Geometry: final body of the model. Coordinates: model frame, mm. A direction names the side the tool comes from. Round coordinates to 2 decimals unless told otherwise and drop trailing zeros. Loops run counter-clockwise (first coordinate to the right, second up) from the corner with the lowest first, then second, coordinate; pieces in that order, holes last. Notation, with made-up numbers: (46.5, -29) - (63.5, -29) arc R31 ccw to (63.5, 6) - close; hole circle Ø11 at (70, -21.75). An arc over 180 degrees is marked (long way). Answer in a Markdown table with one row per item. Add a question column.
from build123d import *

# Parameters (mm, degrees)
SKETCH1_R           = 2.286
SKETCH1_R_2         = 1.181
BOSS_EXTRUDE1_DEPTH = 6.35
SKETCH1_3_R         = 2.286
SKETCH1_3_R_2       = 1.181
CUT_EXTRUDE1_DEPTH  = 3.175


with BuildPart() as part:
    # Sketch1 → Boss-Extrude1 (new body)
    # profile 1 of 3: a face of its own
    with BuildSketch(Plane.XY):
        with BuildLine():
            Line((399.033701588, 239.383854223), (443.033701589, 239.383854223))
            ThreePointArc((443.033701589, 239.383854223), (444.447915151, 239.969640661), (445.033701588, 241.383854223))
            Line((445.033701588, 241.383854223), (445.033701588, 251.383854223))
            ThreePointArc((445.033701588, 251.383854223), (444.447915152, 252.798067786), (443.033701589, 253.383854224))
            Line((443.033701589, 253.383854224), (399.033701588, 253.383854224))
            ThreePointArc((399.033701588, 253.383854224), (397.619488025, 252.798067787), (397.033701588, 251.383854224))
            Line((397.033701588, 251.383854224), (397.033701588, 241.383854224))
            ThreePointArc((397.033701588, 241.383854224), (397.619488025, 239.969640661), (399.033701588, 239.383854223))
        make_face()
        with Locations((403.508701589, 248.883854223)):
            Circle(SKETCH1_R, mode=Mode.SUBTRACT)
        with Locations((413.033701589, 248.883854223)):
            Circle(SKETCH1_R, mode=Mode.SUBTRACT)
        with BuildLine():
            ThreePointArc((421.483701588, 244.433854222), (424.033701588, 241.883854222), (426.583701588, 244.433854222))
            Line((426.583701588, 244.433854222), (426.583701588, 248.333854223))
            ThreePointArc((426.583701588, 248.333854223), (424.033701588, 250.883854223), (421.483701588, 248.333854223))
            Line((421.483701588, 248.333854223), (421.483701588, 244.433854222))
        make_face(mode=Mode.SUBTRACT)
        with BuildLine():
            ThreePointArc((436.483701588, 244.433854222), (439.033701588, 241.883854222), (441.583701588, 244.433854222))
            Line((441.583701588, 244.433854222), (441.583701588, 248.333854223))
            ThreePointArc((441.583701588, 248.333854223), (439.033701588, 250.883854223), (436.483701588, 248.333854223))
            Line((436.483701588, 248.333854223), (436.483701588, 244.433854222))
        make_face(mode=Mode.SUBTRACT)
    # profile 2 of 3: a face of its own
    with BuildSketch(Plane.XY):
        with Locations((413.033701589, 248.883854223)):
            Circle(SKETCH1_R)
        with Locations((413.033701589, 248.883854223)):
            Circle(SKETCH1_R_2, mode=Mode.SUBTRACT)
    # profile 3 of 3: a face of its own
    with BuildSketch(Plane.XY):
        with Locations((403.508701589, 248.883854223)):
            Circle(SKETCH1_R)
        with Locations((403.508701589, 248.883854223)):
            Circle(SKETCH1_R_2, mode=Mode.SUBTRACT)
    extrude(amount=BOSS_EXTRUDE1_DEPTH)

    # Sketch1_3 → Cut-Extrude1 (cut)
    # profile 1 of 2: a face of its own
    with BuildSketch(Plane.XY):
        with Locations((403.508701589, 248.883854223)):
            Circle(SKETCH1_3_R)
        with Locations((403.508701589, 248.883854223)):
            Circle(SKETCH1_3_R_2, mode=Mode.SUBTRACT)
    # profile 2 of 2: a face of its own
    with BuildSketch(Plane.XY):
        with Locations((413.033701589, 248.883854223)):
            Circle(SKETCH1_3_R)
        with Locations((413.033701589, 248.883854223)):
            Circle(SKETCH1_3_R_2, mode=Mode.SUBTRACT)
    extrude(amount=CUT_EXTRUDE1_DEPTH, mode=Mode.SUBTRACT)


solid = part.part
1) Section C-C, the plane y = 242.5. Return the cut outline in (x, z), and give its area (3 significant figures).
2) Material intervals for line 1 along X through (y, z) = (246.75, 6); line 2 along X through (y, z) = (248, 2.75); line 3 along Y through (x, z) = (412, 5.25), sorted ascending. Write a range as from..to.
3) Pull-direction query (Y, two-part tool) for faces 1 (the flat face through (421, 239.384, 3)), 2 (the flat face through (436.484, 246, 3)), 3 (the flat face through (445.034, 246, 3)); classes: pulls with the +Y half, pulls with the -Y half, needs draft (parallel to the pull), parting line crosses it, or undercut.
4) Section B-B, the plane z = 3.75. Return the cut outline in (x, y).
5) Reachability of faces 4 (the flat face through (426.584, 246, 3)), 5 (the flat face through (421, 246, 6.35)), 6 (the cylindrical face through (401.225, 248.984, 1.565)) from +Z, -Z, +X, -X, +Y, -Y: full face, straight path, thin tool, end or side. Return the list, or none.
6) Section A-A, the plane x = 437. Return the cut outline in (y, z), and give its area (3 significant figures).
7) Contact query for a flat-ended pin moving along its axis: pin 1 Ø1.4 at (x, y) = (414, 250) entering from -Z (3 decimals). Output: stop coordinate, or through.
Evaluation:
| question | item | result |
|---|---|---|
| 1 | outline | (397.03, 0) - (422.37, 0) - (422.37, 6.35) - (397.03, 6.35) - close; (425.7, 0) - (437.37, 0) - (437.37, 6.35) - (425.7, 6.35) - close; (440.7, 0) - (445.03, 0) - (445.03, 6.35) - (440.7, 6.35) - close |
| 1 | area | 263 mm² |
| 2 | line 1 | x = 397.03..421.48, 426.58..436.48, 441.58..445.03 |
| 2 | line 2 | x = 397.03..401.4, 405.62..410.93, 415.14..421.48, 426.58..436.48, 441.58..445.03 |
| 2 | line 3 | y = 239.38..248.31, 249.46..253.38 |
| 3 | face 1 | pulls with the -Y half |
| 3 | face 2 | undercut |
| 3 | face 3 | needs draft |
| 4 | outline | (397.03, 241.38) arc R2 ccw to (399.03, 239.38) - (443.03, 239.38) arc R2 ccw to (445.03, 241.38) - (445.03, 251.38) arc R2 ccw to (443.03, 253.38) - (399.03, 253.38) arc R2 ccw to (397.03, 251.38) - close; hole circle Ø2.36 at (403.51, 248.88); hole circle Ø2.36 at (413.03, 248.88); hole (421.48, 244.43) arc R2.55 ccw to (426.58, 244.43) - (426.58, 248.33) arc R2.55 ccw to (421.48, 248.33) - close; hole (436.48, 244.43) arc R2.55 ccw to (441.58, 244.43) - (441.58, 248.33) arc R2.55 ccw to (436.48, 248.33) - close |
| 5 | face 4 | +Z, -Z |
| 5 | face 5 | +Z, +X, -X, +Y, -Y |
| 5 | face 6 | -Z |
| 6 | outline | (239.38, 0) - (242.9, 0) - (242.9, 6.35) - (239.38, 6.35) - close; (249.87, 0) - (253.38, 0) - (253.38, 6.35) - (249.87, 6.35) - close |
| 6 | area | 44.6 mm² |
| 7 | pin 1 | stops at z = 3.175 |
